CAD build for the part. Positions are in the model's coordinates, mm. Face numbers are marked on the shaded views. A direction names the side the tool comes from. Round coordinates to 2 decimals unless told otherwise and drop trailing zeros. Write each loop counter-clockwise with the first axis right and the second up, starting at its lowest first coordinate (ties: lowest second). Pieces come first, ordered by that corner, then holes. Notation, with made-up numbers: (-20.75, -9) -> (-11.75, -9) arc R12 ccw to (-11.75, -5) -> close; hole circle Ø2 at (81, 74.25). An arc over 180 degrees is marked (long way). Put each result on its own line as item: value. Start each with the question number.
1. 3-axis set-ups, long thin cutter, end or side, ignore diameter. For the marked faces 1 and 2: which of +Z, -Z, +X, -X, +Y, -Y reach the whole face in a straight line?
2. Pull direction X, two halves, no side cores. Call the marked faces 3, 4 and 5: pulls with the +X half, pulls with the -X half, needs draft (parallel to the pull), parting line crosses it, or undercut.
3. Saw through at A-A on x = 0. List the corners of the cut face in (y, z), and give its area (3 significant figures).
4. Saw through at D-D on z = 6. List the corners of the cut face in (x, y), and give its area (3 significant figures).
5. Saw through at C-C on y = 32.5. List the corners of the cut face in (x, z).
6. Flat gauge pin, fed straight in: P1, Ø1.5, axis at x = -20.5, z = -21, coming from the +Y side. Where does the tip first touch, or does it go through?
7. Saw through at B-B on z = 34. List the corners of the cut face in (x, y), and give its area (3 significant figures).
8. Drill centre lines: line 1 (X direction, y = 17.5, z = 34); line 2 (Z direction, x = -37.5, y = 37). Where is each one in solid material? Low to high. Write a range as from..to.
Autodesk Inventor part; units mm, degrees
ref_plane "YZ Plane" through (0, 0, 0) normal (1, 0, 0) x (0, 1, 0)
ref_plane "XZ Plane" through (0, 0, 0) normal (0, 1, 0) x (-1, 0, 0)
ref_plane "XY Plane" through (0, 0, 0) normal (0, 0, 1) x (1, 0, 0)
sketch "Sketch1" plane through (0, 0, 0) normal (0, 1, 0) x (-1, 0, 0)
  line L0 (45.9867, -45.9867) -> (-45.9867, -45.9867)
  line L1 (-45.9867, -45.9867) -> (-45.9867, 45.9867)
  line L2 (-45.9867, 45.9867) -> (45.9867, 45.9867)
  line L3 (45.9867, 45.9867) -> (45.9867, -45.9867)
  line L4 (45.9867, -45.9867) -> (-45.9867, 45.9867) construction
  line L5 (-45.9867, -45.9867) -> (45.9867, 45.9867) construction
  point P0 (0, 0)
  dimension "d0" = 91.9734
  dimension "d1" = 91.9734
extrude "Extrusion1" add sketch "Sketch1" along normal blind 2.4892
sketch "Sketch2" plane through (0, 2.4892, 0) normal (0, 1, 0) x (1, 0, 0)
  line L0 (-45.9867, -45.9867) -> (45.9867, -45.9867)
  line L1 (45.9867, 45.9867) -> (-45.9867, 45.9867)
  line L2 (-45.9867, -45.9867) -> (45.9867, -45.9867)
  line L3 (45.9867, -45.9867) -> (45.9867, 45.9867)
  line L4 (45.9867, 45.9867) -> (-45.9867, 45.9867)
  line L5 (-45.9867, 45.9867) -> (-45.9867, -45.9867)
  line L6 (43.4975, -43.4975) -> (-43.4975, 43.4975) construction
  line L7 (-43.4975, -43.4975) -> (43.4975, 43.4975) construction
  line L8 (-45.9867, -45.9867) -> (-36.9951, -45.9867)
  line L9 (-45.9867, -36.9951) -> (-45.9867, -45.9867)
  line L10 (-45.9867, 45.9867) -> (-45.9867, -45.9867)
  line L11 (-45.9867, 45.9867) -> (-36.9951, 45.9867)
  line L12 (-45.9867, 36.9951) -> (-45.9867, 45.9867)
  line L13 (45.9867, 45.9867) -> (36.9951, 45.9867)
  line L14 (45.9867, 36.9951) -> (45.9867, 45.9867)
  line L15 (45.9867, -45.9867) -> (36.9951, -45.9867)
  line L16 (45.9867, -36.9951) -> (45.9867, -45.9867)
  line L17 (-36.9951, -43.4975) -> (-36.9951, -36.9951)
  line L18 (-36.9951, -36.9951) -> (-43.4975, -36.9951)
  line L19 (-43.4975, 36.9951) -> (-36.9951, 36.9951)
  line L20 (-36.9951, 36.9951) -> (-36.9951, 43.4975)
  line L21 (36.9951, 36.9951) -> (43.4975, 36.9951)
  line L22 (36.9951, 43.4975) -> (36.9951, 36.9951)
  line L23 (43.4975, -36.9951) -> (36.9951, -36.9951)
  line L24 (36.9951, -36.9951) -> (36.9951, -43.4975)
  line L25 (-36.9951, -43.4975) -> (36.9951, -43.4975)
  line L26 (43.4975, -36.9951) -> (43.4975, 36.9951)
  line L27 (36.9951, 43.4975) -> (-36.9951, 43.4975)
  line L28 (-43.4975, 36.9951) -> (-43.4975, -36.9951)
  point P0 (0, 0)
  dimension "d4" = 86.995
  dimension "d5" = 86.995
  dimension "d6" = 8.9916
  dimension "d7" = 8.9916
  dimension "d10" = 8.9916
  dimension "d11" = 8.9916
extrude "Extrusion2" add sketch "Sketch2" along normal blind 37.9984
sketch "Sketch3" plane through (0, 2.4892, 0) normal (0, 1, 0) x (1, 0, 0)
  line L0 (25.9969, -22.5044) -> (-25.9969, 22.5044) construction
  line L1 (-25.9969, -22.5044) -> (25.9969, 22.5044) construction
  circle A0 centre (-25.9969, -22.5044) radius 1.9939
  circle A1 centre (-25.9969, 22.5044) radius 1.9939
  circle A2 centre (25.9969, 22.5044) radius 1.9939
  circle A3 centre (25.9969, -22.5044) radius 1.9939
  line L2 (32.9946, -9.9949) -> (-32.9946, 9.9949) construction
  line L3 (-32.9946, -9.9949) -> (32.9946, 9.9949) construction
  circle A4 centre (-32.9946, -9.9949) radius 1.4986
  circle A5 centre (-32.9946, 9.9949) radius 1.4986
  circle A6 centre (32.9946, -9.9949) radius 1.4986
  circle A7 centre (32.9946, 9.9949) radius 1.4986
  circle A8 centre (0, -25.4) radius 2.0828
  circle A9 centre (0, 25.4) radius 2.0828
  point P0 (0, 0)
  dimension "d16" = 51.9938
  dimension "d17" = 45.0088
  dimension "d18" = 3.9878
  dimension "d19" = 3.9878
  dimension "d20" = 3.9878
  dimension "d21" = 3.9878
  dimension "d22" = 65.9892
  dimension "d23" = 19.9898
  dimension "d24" = 2.9972
  dimension "d25" = 2.9972
  dimension "d26" = 2.9972
  dimension "d27" = 2.9972
  dimension "d30" = 4.1656
  dimension "d31" = 4.1656
extrude "Extrusion3" cut sketch "Sketch3" against normal through all
sketch "Sketch4" plane through (-43.4975, 2.4892, 36.9951) normal (1, 0, 0) x (0, 0, -1)
  line L0 (0, 0) -> (0, 37.9984)
  line L1 (0, 19.05) -> (9.4996, 19.05)
  line L2 (0, 19.05) -> (9.4996, 19.05) construction
  line L3 (9.4996, 19.05) -> (30.7594, 19.05)
  line L4 (30.7594, 19.05) -> (45.4406, 19.05)
  circle A0 centre (30.7594, 19.05) radius 3.175
  circle A1 centre (45.4406, 19.05) radius 3.175
  point P0 (36.9951, -2.4892)
  point P1 (73.9902, 0)
  dimension "d44" = 9.4996
  dimension "d45" = 0
  dimension "d46" = 21.2598
  dimension "d47" = 14.6812
  dimension "d48" = 6.35
  dimension "d49" = 6.35
extrude "Extrusion4" cut sketch "Sketch4" against normal through all
sketch "Sketch5" plane through (43.4975, 2.4892, -36.9951) normal (-1, 0, 0) x (0, 0, 1)
  line L0 (73.9902, 0) -> (73.9902, 37.9984)
  line L1 (73.9902, 19.05) -> (64.4906, 19.05)
  line L2 (64.4906, 19.05) -> (43.2308, 19.05)
  line L3 (43.2308, 19.05) -> (28.5496, 19.05)
  circle A0 centre (43.2308, 19.05) radius 3.175
  circle A1 centre (28.5496, 19.05) radius 3.175
  point P0 (36.9951, -2.4892)
  point P1 (0, 37.9984)
  dimension "d50" = 9.4996
  dimension "d51" = 21.2598
  dimension "d52" = 14.6812
  dimension "d53" = 6.35
  dimension "d54" = 6.35
extrude "Extrusion5" cut sketch "Sketch5" against normal through all
properties part number "546-1590YFLBK-ADL5534"
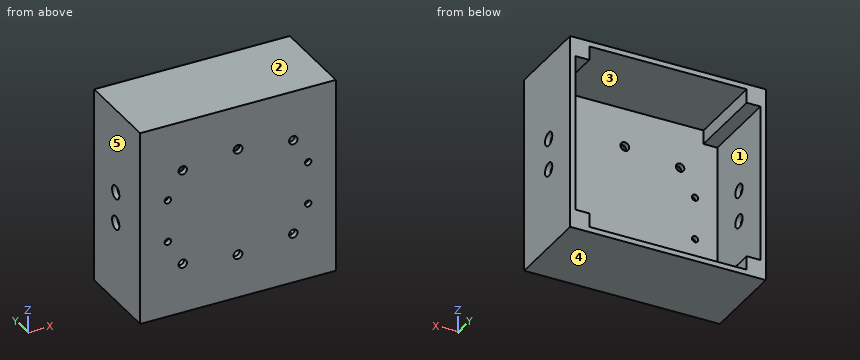
Return value:
1. face 1: +Y
1. face 2: +Z, +X, -X, +Y, -Y
2. face 3: undercut
2. face 4: needs draft
2. face 5: pulls with the -X half
3. outline: (0, -45.99) -> (40.49, -45.99) -> (40.49, -43.5) -> (2.49, -43.5) -> (2.49, -27.48) -> (0, -27.48) -> close; (0, -23.32) -> (2.49, -23.32) -> (2.49, 23.32) -> (0, 23.32) -> close; (0, 27.48) -> (2.49, 27.48) -> (2.49, 43.5) -> (40.49, 43.5) -> (40.49, 45.99) -> (0, 45.99) -> close
3. area: 397 mm^2
4. outline: (-45.99, 0) -> (45.99, 0) -> (45.99, 18.37) -> (43.5, 18.37) -> (43.5, 2.49) -> (-43.5, 2.49) -> (-43.5, 18.37) -> (-45.99, 18.37) -> close; (-45.99, 24.71) -> (-43.5, 24.71) -> (-43.5, 40.49) -> (-45.99, 40.49) -> close; (43.5, 24.71) -> (45.99, 24.71) -> (45.99, 40.49) -> (43.5, 40.49) -> close
4. area: 387 mm^2
5. outline: (-45.99, -45.99) -> (45.99, -45.99) -> (45.99, 45.99) -> (-45.99, 45.99) -> close; hole (-43.5, -37) -> (-37, -37) -> (-37, -43.5) -> (37, -43.5) -> (37, -37) -> (43.5, -37) -> (43.5, 37) -> (37, 37) -> (37, 43.5) -> (-37, 43.5) -> (-37, 37) -> (-43.5, 37) -> close
6. P1: stops at y = 2.49
7. outline: (-45.99, 0) -> (45.99, 0) -> (45.99, 40.49) -> (43.5, 40.49) -> (43.5, 2.49) -> (-43.5, 2.49) -> (-43.5, 40.49) -> (-45.99, 40.49) -> close
7. area: 418 mm^2
8. line 1: x = -45.99..-43.5, 43.5..45.99
8. line 2: z = -45.99..-37, 37..45.99
